Build history of the part. All positions in model axes, mm. Face numbers are marked on the shaded views. Give positions to 0.01 mm unless a question says otherwise; leave off trailing zeros. Loops run counter-clockwise (first coordinate to the right, second up) from the corner with the lowest first, then second, coordinate; pieces in that order, holes last.
1) Band-saw the part on A-A on z = 0. List the corners of the cut face in (x, y).
2) Two-plate mould, pull along Z, no slides. Class the marked faces 1, 2 and 3: +Z half, -Z half, draft (parallel to the pull), parting line (faces both ways), or undercut.
3) Wall check: line 1 (Z direction, x = 0, y = 35.7); line 2 (X direction, y = 33.6, z = 0); line 3 (X direction, y = 12, z = -9). Give the ranges that are in metal, low to high.
4) Band-saw the part on D-D on x = 16.5. List the corners of the cut face in (y, z).
5) Flat gauge pins, fed straight in: P1, Ø6, axis at y = 31.5, z = -5.5, coming from the +X side; P2, Ø1, axis at y = 5.5, z = -7.5, coming from the -X side; P3, Ø3, axis at x = 0, z = 0.5, coming from the +Y side. Where does each tip first touch, or does it go through?
6) Band-saw the part on C-C on z = -8.25. List the corners of the cut face in (x, y), then the cut area to 3 significant figures.
7) Band-saw the part on B-B on x = 0. List the corners of the cut face in (y, z).
```python
from build123d import *

# Parameters (mm, degrees)
SKETCH1_W           = 40
SKETCH1_H           = 20
BOSS_EXTRUDE1_DEPTH = 37
FILLET1_R           = 5
SKETCH2_R           = 3
CUT_EXTRUDE1_DEPTH  = 5


with BuildPart() as part:
    # Sketch1 → Boss-Extrude1 (new body)
    with BuildSketch(Plane(origin=(0, 0, 0), x_dir=(1, 0, 0), z_dir=(0, 1, 0))):
        Rectangle(SKETCH1_W, SKETCH1_H)
    extrude(amount=BOSS_EXTRUDE1_DEPTH)

    # Fillet1
    fillet1_edges = [part.edges().sort_by_distance(p)[0] for p in [
        (20, 18.5, 10),
        (-20, 18.5, 10),
        (-20, 18.5, -10),
        (20, 18.5, -10),
    ]]
    fillet(fillet1_edges, radius=FILLET1_R)

    # Sketch2 → Cut-Extrude1 (cut)
    with BuildSketch(Plane(origin=(0, 37, 0), x_dir=(1, 0, 0), z_dir=(0, 1, 0))):
        Circle(SKETCH2_R)
    extrude(amount=-CUT_EXTRUDE1_DEPTH, mode=Mode.SUBTRACT)


solid = part.part
```
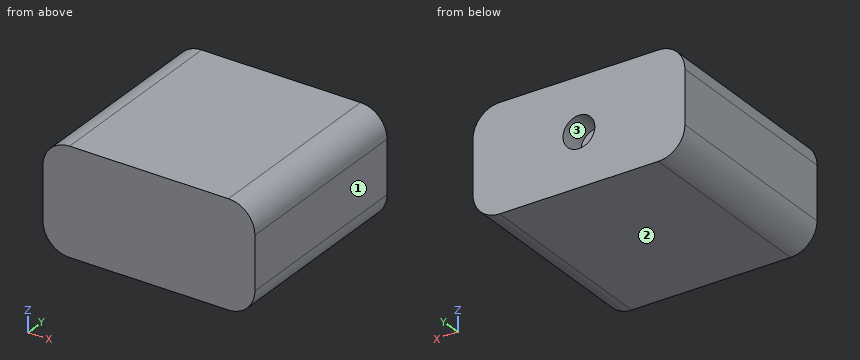
Findings below:
1. outline: (-20, 0) - (20, 0) - (20, 37) - (3, 37) - (3, 32) - (-3, 32) - (-3, 37) - (-20, 37) - close
2. face 1: draft
2. face 2: -Z half
2. face 3: undercut
3. line 1: z = -10 to -3, 3 to 10
3. line 2: x = -20 to -3, 3 to 20
3. line 3: x = -18 to 18
4. outline: (0, -9.77) - (37, -9.77) - (37, 9.77) - (0, 9.77) - close
5. P1: stops at x = 20
5. P2: stops at x = -19.58
5. P3: stops at y = 32
6. outline: (-18.8, 0) - (18.8, 0) - (18.8, 37) - (-18.8, 37) - close
6. area: 1,390 mm2
7. outline: (0, -10) - (37, -10) - (37, -3) - (32, -3) - (32, 3) - (37, 3) - (37, 10) - (0, 10) - close
